Part model, mm, in its own coordinate system. A direction names the side the tool comes from. Give positions to 0.01 mm unless a question says otherwise; leave off trailing zeros. Write each loop counter-clockwise with the first axis right and the second up, starting at its lowest first coordinate (ties: lowest second). Pieces come first, ordered by that corner, then holes. Notation, with made-up numbers: M 63.5,-29 L 112.5,-29 A10 ccw 112.5,-21 Z; hole C 79,18 d2. An arc over 180 degrees is marked long. Answer as CSV lines item,"result". Start each with the question number.
Item 1: Band-saw the part on B-B, the plane y = 3. List the corners of the cut face in (x, z).
Item 2: Band-saw the part on C-C, the plane x = 16. List the corners of the cut face in (y, z).
Item 3: 3-axis set-ups, long thin cutter, end or side, ignore diameter. For faces 1 (the cylindrical face through (-23.626, -4.71, 2.535)), 2 (the flat face through (20, -15, 2)), 3 (the flat face through (-19, 20, 2)): which of +Z, -Z, +X, -X, +Y, -Y reach the whole face in a straight line?
Item 4: Pin check, flat tips, straight feed: pin 1 (2.5 mm diameter, centred on x = -16, y = -16, fed in from +Z); pin 2 (3 mm diameter, centred on x = -22, y = 16, fed in from -Z); pin 3 (1.5 mm diameter, centred on x = -12, z = 0.5, fed in from -Y); pin 4 (2.5 mm diameter, centred on y = 14, z = 3, fed in from +X). Stop position of each tip, or through.
Item 5: Band-saw the part on D-D, the plane z = 2.75. Count the separate pieces of the cut face and the enclosed holes in it, then the cut area to 3 significant figures.
Item 6: Wall check: L1, parallel to Y at x = -33.5, z = 2.25; L2, parallel to Y at x = 16, z = 2.25; L3, parallel to X at y = -15, z = 1.7. Give the ranges that are in metal, low to high. Write a range as from..to.
Item 7: Two-plate mould, pull along X, no slides. Class faces 4 (the flat face through (-11, -20, 2)), 5 (the cylindrical face through (-16.958, 16.879, 2.465)), 6 (the cylindrical face through (9.3, -20.1, 2.5)), 7 (the cylindrical face through (-22.65, 8.97, 2.46)): +X half, -X half, draft (parallel to the pull), parting line (faces both ways), or undercut.
Item 8: Band-saw the part on A-A, the plane x = 7.5. List the corners of the cut face in (y, z).
from build123d import *

# Parameters (mm, degrees)
SKETCH1_R           = 19
SKETCH1_R_2         = 1.6
SKETCH1_R_3         = 1.3
BOSS_EXTRUDE1_DEPTH = 5
FILLET1_R           = 12
FILLET3_R           = 12
FILLET4_R           = 1
FILLET5_R           = 6
SKETCH6_R           = 1.25
BOSS_EXTRUDE3_DEPTH = 5
FILLET6_R           = 10
FILLET8_R           = 7


with BuildPart() as part:
    # Sketch1 → Boss-Extrude1 (new body)
    with BuildSketch(Plane.XY):
        with BuildLine():
            Line((-37.3, -16.9), (-37.3, -26.9))
            ThreePointArc((-37.3, -26.9), (-35.439240178, -30.051990419), (-31.780531331, -29.945593543))
            Line((-31.780531331, -29.945593543), (-16, -20))
            Line((-16, -20), (-9.16515139, -20))
            ThreePointArc((-9.16515139, -20), (0, -22), (9.16515139, -20))
            Line((9.16515139, -20), (20, -20))
            Line((20, -20), (20, -9.16515139))
            ThreePointArc((20, -9.16515139), (22, 0), (20, 9.16515139))
            Line((20, 9.16515139), (20, 20))
            Line((20, 20), (9.16515139, 20))
            ThreePointArc((9.16515139, 20), (0, 22), (-9.16515139, 20))
            Line((-9.16515139, 20), (-20, 20))
            Line((-20, 20), (-20, 9.16515139))
            ThreePointArc((-20, 9.16515139), (-21.885463921, 2.241978803), (-21.442870984, -4.91968332))
            Line((-21.442870984, -4.91968332), (-35.619468669, -13.854406457))
            ThreePointArc((-35.619468669, -13.854406457), (-36.851990419, -15.160759822), (-37.3, -16.9))
        make_face()
        Circle(SKETCH1_R, mode=Mode.SUBTRACT)
        with Locations((-33.7, -16.9)):
            Circle(SKETCH1_R_2, mode=Mode.SUBTRACT)
        with Locations((-33.7, -26.9)):
            Circle(SKETCH1_R_2, mode=Mode.SUBTRACT)
        with Locations((-16, 16)):
            Circle(SKETCH1_R_3, mode=Mode.SUBTRACT)
        with Locations((16, 16)):
            Circle(SKETCH1_R_3, mode=Mode.SUBTRACT)
        with Locations((16, -16)):
            Circle(SKETCH1_R_2, mode=Mode.SUBTRACT)
        with Locations((-16, -16)):
            Circle(SKETCH1_R_2, mode=Mode.SUBTRACT)
    extrude(amount=BOSS_EXTRUDE1_DEPTH)

    # Fillet1
    fillet1_edges = [part.edges().sort_by_distance(p)[0] for p in [
        (-21.442870984, -4.91968332, 2.5),
    ]]
    fillet(fillet1_edges, radius=FILLET1_R)

    # Fillet3
    fillet3_edges = [part.edges().sort_by_distance(p)[0] for p in [
        (-16, -20, 2.5),
    ]]
    fillet(fillet3_edges, radius=FILLET3_R)

    # Fillet4
    fillet4_edges = [part.edges().sort_by_distance(p)[0] for p in [
        (20, 20, 2.5),
        (20, -20, 2.5),
    ]]
    fillet(fillet4_edges, radius=FILLET4_R)

    # Fillet5
    fillet5_edges = [part.edges().sort_by_distance(p)[0] for p in [
        (9.16515139, -20, 2.5),
        (-9.16515139, -20, 2.5),
        (20, 9.16515139, 2.5),
        (20, -9.16515139, 2.5),
    ]]
    fillet(fillet5_edges, radius=FILLET5_R)

    # Sketch6 → Boss-Extrude3 (add)
    with BuildSketch(Plane(origin=(0, 0, 0), x_dir=(-1, 0, 0), z_dir=(0, 0, -1))):
        with BuildLine():
            Line((22, 20), (20, 20))
            Line((20, 20), (20, 12))
            Line((20, 12), (22, 12))
            Line((22, 12), (28, 12))
            ThreePointArc((28, 12), (32, 16), (28, 20))
            Line((28, 20), (22, 20))
        make_face()
        with Locations((22, 16)):
            Circle(SKETCH6_R, mode=Mode.SUBTRACT)
        with Locations((28, 16)):
            Circle(SKETCH6_R, mode=Mode.SUBTRACT)
    extrude(amount=-BOSS_EXTRUDE3_DEPTH)

    # Fillet6
    # the kernel refuses this fillet: 10 mm, written as the material it adds along each edge
    with BuildSketch(Plane(origin=(-20, 12, 0), x_dir=(0, -1, 0), z_dir=(0, 0, 1))) as fillet6_piece_1:
        with BuildLine():
            CenterArc((10, -6.975715416), FILLET6_R, 135.767508297, 44.232491703)
            Line((0, -6.975715416), (-0.2, -6.975715416))
            Line((-0.2, -6.975715416), (-0.2, 0))
            Line((-0.2, 0), (0, 0.2))
            ThreePointArc((0, 0.2), (1.417424305, 0.2), (2.691545582, 0.139514308))
            Line((2.691545582, 0.139514308), (2.83484861, 0))
        make_face()
    extrude(amount=5)

    # Fillet8
    # the kernel refuses this fillet: 7 mm, written as the material it adds along each edge
    with BuildSketch(Plane(origin=(-20, 9.16515139, 0), x_dir=(-0.9264219176463756, 0.3764869592753673, 0), z_dir=(0, 0, 1))) as fillet8_piece_1:
        with BuildLine():
            CenterArc((6.404489612, 6.90896616), FILLET8_R, 191.835369606, 87.415058428)
            ThreePointArc((-0.446697133, 5.473264176), (-0.051904318, 2.750624406), (0, 0))
            ThreePointArc((0, 0), (3.764869593, -0.735780824), (7.529739186, 0))
        make_face()
    extrude(amount=5)


solid = part.part
Output:
1,outline,"M -21.79,0 L -18.76,0 L -18.76,5 L -21.79,5 Z; M 18.76,0 L 21.79,0 L 21.79,5 L 18.76,5 Z"
2,outline,"M -20,0 L -17.6,0 L -17.6,5 L -20,5 Z; M -14.4,0 L -10.25,0 L -10.25,5 L -14.4,5 Z; M 10.25,0 L 14.7,0 L 14.7,5 L 10.25,5 Z; M 17.3,0 L 20,0 L 20,5 L 17.3,5 Z"
3,face 1,"+Z, -Z, -X"
3,face 2,"+Z, -Z, +X, -Y"
3,face 3,"+Z, -Z, -X, +Y"
4,pin 1,"through"
4,pin 2,"z = 0"
4,pin 3,"y = -20"
4,pin 4,"x = 20"
5,separate pieces,"1"
5,enclosed holes,"9"
5,area,"938 mm²"
6,L1,"-30.49..-28.49, -25.31..-18.49, -15.31..-12.52"
6,L2,"-20..-17.6, -14.4..-10.25, 10.25..14.7, 17.3..20"
6,L3,"-36.76..-17.25, -14.75..-11.66, 11.66..14.75, 17.25..20"
7,face 4,"undercut"
7,face 5,"undercut"
7,face 6,"+X half"
7,face 7,"-X half"
8,outline,"M -20.68,0 L -17.46,0 L -17.46,5 L -20.68,5 Z; M 17.46,0 L 20.68,0 L 20.68,5 L 17.46,5 Z"
